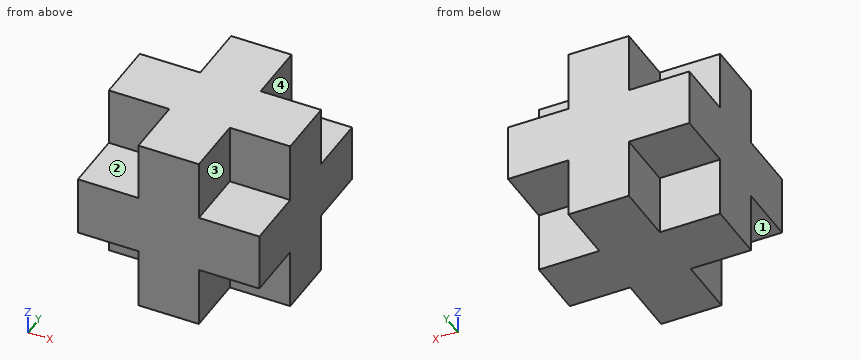
```python
from build123d import *

# Parameters (mm, degrees)
F0_W      = 152.4
F0_H      = 149.9905144195
F1_DEPTH  = 152.4
F2_W      = 50.8
F2_H      = 49.1875803169
F3_DEPTH  = 50.8
F4_W      = 50.8
F4_H      = 50.3492622576
F5_DEPTH  = 50.8
F6_W      = 50.8
F6_H      = 50.8
F7_DEPTH  = 343
F8_W      = 50.8
F8_H      = 50.8
F9_DEPTH  = 50.8
F10_W     = 50.8
F10_H     = 50.8
F11_DEPTH = 50.8
F12_W     = 50.8
F12_H     = 50.8
F13_DEPTH = 50.8


# Not quite as in the source:
# - an extrude ends at something that could not be found from the text; its depth is read off the source's solid
# - a feature names something its author has since deleted; it is built from what else it names


with BuildPart() as f1:
    # F0 (on Front) → F1 (new body)
    with BuildSketch(Plane.XZ):
        with Locations((3.4536700696, 3.1658634543)):
            Rectangle(F0_W, F0_H)
    extrude(amount=F1_DEPTH)

    # F2 (on face) → F3 (cut)
    with BuildSketch(Plane.XZ.offset(152.4)):
        with Locations((-47.3463299304, 53.5673305057)):
            Rectangle(F2_W, F2_H)
    extrude(amount=-F3_DEPTH, mode=Mode.SUBTRACT)

    # F4 (on face) → F5 (cut)
    with BuildSketch(Plane.XZ.offset(152.4)):
        with Locations((54.2536700696, 52.9864895353)):
            Rectangle(F4_W, F4_H)
    extrude(amount=-F5_DEPTH, mode=Mode.SUBTRACT)

    # F6 (on face) → F7 (cut, through all)
    with BuildSketch(Plane.XZ.offset(152.4)):
        with Locations((-47.3463299304, -46.4293937554)):
            Rectangle(F6_W, F6_H)
    extrude(amount=F7_DEPTH, mode=Mode.SUBTRACT)

    # F8 (on face) → F9 (cut)
    with BuildSketch(Plane(origin=(0, 0, 0), x_dir=(-1, 0, 0), z_dir=(0, 1, 0))):
        with Locations((-54.2536700696, -46.4293937554)):
            Rectangle(F8_W, F8_H)
        with Locations((47.3463299304, -46.4293937554)):
            Rectangle(F8_W, F8_H)
    extrude(amount=-F9_DEPTH, mode=Mode.SUBTRACT)

    # F10 (on face) → F11 (cut)
    with BuildSketch(Plane(origin=(0, 0, -71.8293937554), x_dir=(1, 0, 0), z_dir=(0, 0, -1))):
        with Locations((-47.3463299304, 127)):
            Rectangle(F10_W, F10_H)
        with Locations((54.2536700696, 127)):
            Rectangle(F10_W, F10_H)
    extrude(amount=-F11_DEPTH, mode=Mode.SUBTRACT)

    # F12 (on face) → F13 (cut)
    with BuildSketch(Plane.XY.offset(78.1611206641)):
        with Locations((-47.3463299304, -25.4)):
            Rectangle(F12_W, F12_H)
        with Locations((54.2536700696, -25.4)):
            Rectangle(F12_W, F12_H)
    extrude(amount=-F13_DEPTH, mode=Mode.SUBTRACT)


solid = f1.part
```
Can you work these out from the model? Positions are in its coordinate system, mm. Face numbers are marked on the shaded views. A direction names the side the tool comes from. Coordinates: 2 decimals unless noted, no trailing zeros. Loops run counter-clockwise (first coordinate to the right, second up) from the corner with the lowest first, then second, coordinate; pieces in that order, holes last.
1) Imagine slicing it at B-B on z = 56. List the corners of the cut face in (x, y) for me, plus the area to 3 significant figures.
2) I need wall thicknesses on probe 1 along X at (y, z) = (-7.5, 63); probe 2 along Y at (x, z) = (-54, -64); probe 3 along Z at (x, y) = (-58, -34.5). Which ranges of each line are inside material? Lowest first, please.
3) Imagine slicing it at A-A on x = 36. List the corners of the cut face in (y, z) for me, plus the area to 3 significant figures.
4) Which directions (+Z, -Z, +X, -X, +Y, -Y) give clear straight access to the entire face, cutting with the end or side of a thin tool? Please do the marked faces 1, 2, 3 and 4.
5) For pin 1 (15 mm diameter, centred on y = -35, z = -49.5, fed in from -X); pin 2 (15 mm diameter, centred on y = -138.5, z = -46, fed in from +X); pin 3 (4 mm diameter, centred on x = 59.5, z = -36, fed in from -Y); pin 4 (10 mm diameter, centred on x = -23, y = -17.5, fed in from +Z), each with a flat end and sliding along its axis, tell me the tip position at first contact or that it passes through.
Completed:
1. outline: (-72.75, -101.6) - (-21.95, -101.6) - (-21.95, -152.4) - (28.85, -152.4) - (28.85, -101.6) - (79.65, -101.6) - (79.65, -50.8) - (28.85, -50.8) - (28.85, 0) - (-21.95, 0) - (-21.95, -50.8) - (-72.75, -50.8) - close
1. area: 12,900 mm2
2. probe 1: x = -21.95 to 28.85
2. probe 2: y = -101.6 to -50.8
2. probe 3: z = -21.03 to 27.36
3. outline: (-152.4, -21.03) - (-101.6, -21.03) - (-101.6, -71.83) - (-50.8, -71.83) - (-50.8, -21.03) - (0, -21.03) - (0, 27.36) - (-50.8, 27.36) - (-50.8, 78.16) - (-101.6, 78.16) - (-101.6, 27.81) - (-152.4, 27.81) - close
3. area: 12,600 mm2
4. face 1: -Z, -X, -Y
4. face 2: +Z, -X, -Y
4. face 3: +Z, +X, -Y
4. face 4: +Z, +X, +Y
5. pin 1: stops at x = -21.95
5. pin 2: stops at x = 28.85
5. pin 3: stops at y = -101.6
5. pin 4: stops at z = 78.16
